Geometry check sheet. Reference: the model listing, model coordinates, mm. Give positions to 0.01 mm unless a question says otherwise; leave off trailing zeros. Write each loop counter-clockwise with the first axis right and the second up, starting at its lowest first coordinate (ties: lowest second). Pieces come first, ordered by that corner, then holes. Notation, with made-up numbers: (11, -23) -> (43, -23) arc R24 ccw to (43, -6) -> close; hole circle Ø7 at (17.5, 20). An arc over 180 degrees is marked (long way). Write item = value, one per line. Start each with the question number.
1. Cross-section at B-B, the plane x = 17.5. Record the cut outline in (y, z).
2. Thickness scan on line 1 along Y through (x, z) = (-6.5, 6.5); line 2 along Y through (x, z) = (-11, 11.5). Record the ranges inside material, lowest first.
3. Depth check by flat-ended pin: P1, Ø5, axis at x = 28.5, z = -5.5, coming from the +Y side; P2, Ø3, axis at x = -22.5, z = -6, coming from the +Y side (3 decimals); P3, Ø5, axis at x = -3.5, z = -4.5, coming from the +Y side. Enter the tip coordinate at first touch or a pass-through.
4. Cross-section at A-A, the plane z = 12. Record the cut outline in (x, y), plus the area to 3 significant figures.
```python
from build123d import *

# Parameters (mm, degrees)
SKETCH1_W           = 88.9
SKETCH1_H           = 38.1
BOSS_EXTRUDE1_DEPTH = 2032
CUT_EXTRUDE2_DEPTH  = 39.1
CUT_EXTRUDE3_DEPTH  = 39.1


with BuildPart() as part:
    # Sketch1 → Boss-Extrude1 (new body)
    with BuildSketch(Plane(origin=(0, 0, 0), x_dir=(1, 0, 0), z_dir=(0, 1, 0))):
        Rectangle(SKETCH1_W, SKETCH1_H)
    extrude(amount=BOSS_EXTRUDE1_DEPTH)

    # Sketch2 → Cut-Extrude2 (cut, through all)
    with BuildSketch(Plane.XY.offset(19.05)):
        Polygon((-44.45, 1806.041104583), (-6.454118941, 1854.591397047), (44.45, 1814.753390919), (44.45, 2032), (-44.45, 2032), align=None)
    extrude(amount=-CUT_EXTRUDE2_DEPTH, mode=Mode.SUBTRACT)

    # Sketch3 → Cut-Extrude3 (cut, through all)
    with BuildSketch(Plane.XY.offset(19.05)):
        Polygon((44.45, 65.04415198), (-6.454118941, 0), (-44.45, 29.735906916), (-64.239470553, 4.449361209), (31.244243748, -54.430099769), (82.106502152, 35.573845948), align=None)
    extrude(amount=-CUT_EXTRUDE3_DEPTH, mode=Mode.SUBTRACT)


solid = part.part
```
Answers:
q1.outline = (30.61, -19.05) -> (1835.84, -19.05) -> (1835.84, 19.05) -> (30.61, 19.05) -> close
q2.line_1 = 0.04 to 1854.53
q2.line_2 = 3.56 to 1848.78
q3.P1 = 1829.19
q3.P2 = 1836.005
q3.P3 = 1854.24
q4.outline = (-44.45, 29.74) -> (-6.45, 0) -> (44.45, 65.04) -> (44.45, 1814.75) -> (-6.45, 1854.59) -> (-44.45, 1806.04) -> close
q4.area = 161,000 mm^2
